from build123d import *

# Parameters (mm, degrees)
F0_W     = 370
F0_H     = 65
F0_R     = 3
F1_DEPTH = 25
F3_DEPTH = 25
F4_R     = 8.382557
F4_R_2   = 8.524465
F5_DEPTH = 25


with BuildPart() as f1:
    # F0 (on Front) → F1 (new body)
    with BuildSketch(Plane.XZ):
        Rectangle(F0_W, F0_H)
        with Locations((-174.5, -22.5)):
            Circle(F0_R, mode=Mode.SUBTRACT)
        with BuildLine():
            ThreePointArc((-128.054669, 9.662031), (-116.5, 18.423264), (-104.945331, 9.662031))
            ThreePointArc((-104.945331, 9.662031), (-103.594078, 6.750238), (-101.389864, 4.416603))
            ThreePointArc((-101.389864, 4.416603), (-96.291745, -12.308896), (-110.5, -22.5))
            Line((-110.5, -22.5), (-122.5, -22.5))
            ThreePointArc((-122.5, -22.5), (-136.708255, -12.308896), (-131.610136, 4.416603))
            ThreePointArc((-131.610136, 4.416603), (-129.405922, 6.750238), (-128.054669, 9.662031))
        make_face(mode=Mode.SUBTRACT)
        with BuildLine():
            ThreePointArc((-48.054669, 9.662031), (-36.5, 18.423264), (-24.945331, 9.662031))
            ThreePointArc((-24.945331, 9.662031), (-23.594078, 6.750238), (-21.389864, 4.416603))
            ThreePointArc((-21.389864, 4.416603), (-16.291745, -12.308896), (-30.5, -22.5))
            Line((-30.5, -22.5), (-42.5, -22.5))
            ThreePointArc((-42.5, -22.5), (-56.708255, -12.308896), (-51.610136, 4.416603))
            ThreePointArc((-51.610136, 4.416603), (-49.405922, 6.750238), (-48.054669, 9.662031))
        make_face(mode=Mode.SUBTRACT)
        with Locations((13, -22.5)):
            Circle(F0_R, mode=Mode.SUBTRACT)
        with Locations((175.5, -22.5)):
            Circle(F0_R, mode=Mode.SUBTRACT)
        with Locations((-99, 26.5)):
            Circle(F0_R, mode=Mode.SUBTRACT)
        with Locations((-54, 26.5)):
            Circle(F0_R, mode=Mode.SUBTRACT)
        with Locations((81, 26.5)):
            Circle(F0_R, mode=Mode.SUBTRACT)
        with Locations((126, 26.5)):
            Circle(F0_R, mode=Mode.SUBTRACT)
    extrude(amount=F1_DEPTH)

    # F2 (on face) → F3 (cut)
    with BuildSketch(Plane.XZ.offset(25)):
        with BuildLine():
            ThreePointArc((128.389864, 4.416603), (123.291745, -12.308896), (137.5, -22.5))
            Line((137.5, -22.5), (149.5, -22.5))
            ThreePointArc((149.5, -22.5), (163.708255, -12.308896), (158.610136, 4.416603))
            ThreePointArc((158.610136, 4.416603), (156.405922, 6.750238), (155.054669, 9.662031))
            ThreePointArc((155.054669, 9.662031), (143.5, 18.423264), (131.945331, 9.662031))
            ThreePointArc((131.945331, 9.662031), (130.594078, 6.750238), (128.389864, 4.416603))
        make_face()
        with BuildLine():
            Line((57.5, -22.5), (69.5, -22.5))
            ThreePointArc((69.5, -22.5), (83.708255, -12.308896), (78.610136, 4.416603))
            ThreePointArc((78.610136, 4.416603), (76.405922, 6.750238), (75.054669, 9.662031))
            ThreePointArc((75.054669, 9.662031), (63.5, 18.423264), (51.945331, 9.662031))
            ThreePointArc((51.945331, 9.662031), (50.594078, 6.750238), (48.389864, 4.416603))
            ThreePointArc((48.389864, 4.416603), (43.291745, -12.308896), (57.5, -22.5))
        make_face()
    extrude(amount=-F3_DEPTH, mode=Mode.SUBTRACT)

    # F4 (on face) → F5 (cut)
    with BuildSketch(Plane.XZ.offset(25)):
        with Locations((-166.68272, 14.735676)):
            Circle(F4_R)
        with Locations((-154.677153, -10.931376)):
            Circle(F4_R_2)
    extrude(amount=-F5_DEPTH, mode=Mode.SUBTRACT)


solid = f1.part
Source: CAD feature listing. Evaluate the final solid. Frame: model axes, mm. A direction names the side the tool comes from. Give positions to 0.01 mm unless a question says otherwise; leave off trailing zeros. Write each loop counter-clockwise with the first axis right and the second up, starting at its lowest first coordinate (ties: lowest second). Pieces come first, ordered by that corner, then holes. Notation, with made-up numbers: (-17.75, 15) -> (36.25, 15) arc R28 cw to (36.25, 33) -> close; hole circle Ø7 at (77, 23.5). An arc over 180 degrees is marked (long way). Return JSON: item names as keys, results as strings. Group by question number.
1. Section A-A, the plane x = -38.5. Output: boundary loops of the cut face in (y, z), then the cut area to 3 significant figures.
2. Section B-B, the plane y = -7.75. Count the separate pieces of the cut face and the enclosed holes in it, then the cut area to 3 significant figures.
3. Pin query (flat end, axial travel): pin 1 Ø5 at (x, z) = (-174.5, -22.5) entering from -Y. Return the tip coordinate at first contact, or that it passes through.
4. Mould query, pull axis Z, two halves, no side actions, for faces 1 (the face through (-3, 0, 0)), 2 (the face through (-3, -12, -32.5)), 3 (the face through (78, -12.3, 26.6)). Classes: +Z half, -Z half, draft (parallel to the pull), parting line (faces both ways), or undercut.
5. Material intervals for line 1 (X direction, y = -13, z = 8); line 2 (Z direction, x = -99, y = -9.5); line 3 (X direction, y = -1.25, z = -12), sorted ascending. Write a range as from..to.
6. Access query for faces 4 (the face through (185, -12, 0)), 5 (the face through (-16.21, -12.32, -12.06)). Directions: +Z, -Z, +X, -X, +Y, -Y. A direction counts if a zero-diameter tool reaches every point of the face in a straight line with its end or side. Return the directions, or none.
Determined:
{
 "1": {"outline": "(-25, -32.5) -> (0, -32.5) -> (0, -22.5) -> (-25, -22.5) -> close; (-25, 18.26) -> (0, 18.26) -> (0, 32.5) -> (-25, 32.5) -> close", "area": "606 mm2"},
 "2": {"separate pieces": "1", "enclosed holes": "13", "area": "18,300 mm2"},
 "3": {"pin 1": "passes through"},
 "4": {"face 1": "draft", "face 2": "-Z half", "face 3": "undercut"},
 "5": {"line 1": "x = -185..-171.67, -161.69..-128.68, -104.32..-48.68, -24.32..51.32, 75.68..131.32, 155.68..185", "line 2": "z = -32.5..-17.13, 2.13..23.5, 29.5..32.5", "line 3": "x = -185..-163.13, -146.22..-136.81, -96.19..-56.81, -16.19..43.19, 83.81..123.19, 163.81..185"},
 "6": {"face 4": "+Z, -Z, +X, +Y, -Y", "face 5": "+Y, -Y"}
}
